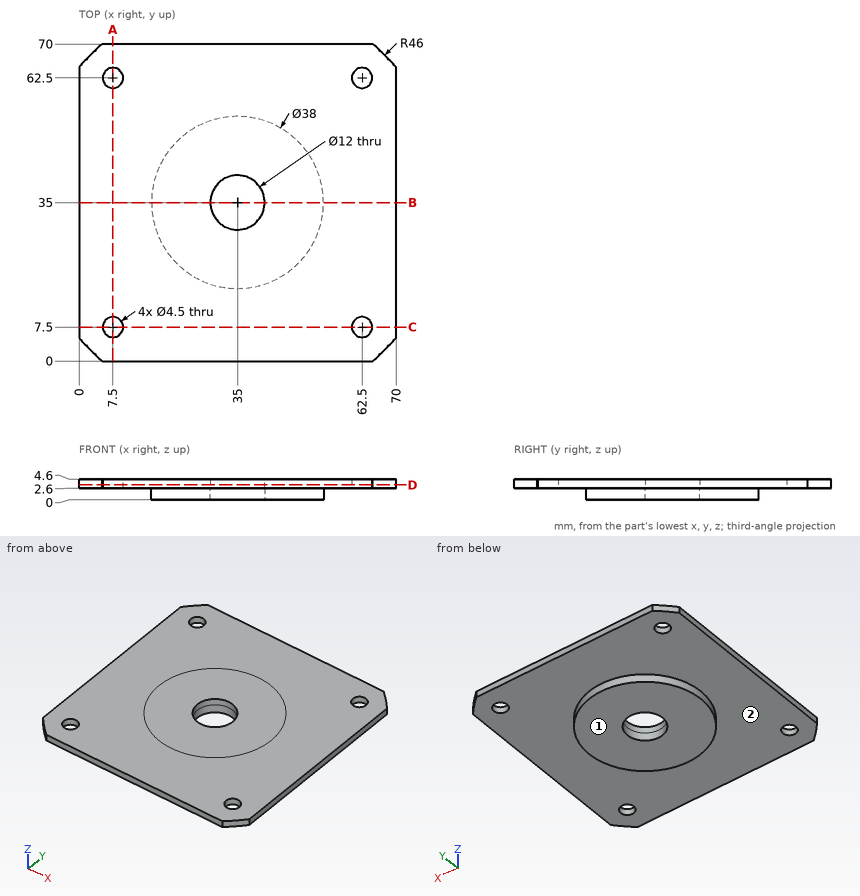
Design review of the part shown in the three views and the two pictorial views. Dimensions are in mm from the part's minimum x, y and z. A direction names the side the tool comes from. Round coordinates to 2 decimals unless told otherwise and drop trailing zeros. Write each loop counter-clockwise with the first axis right and the second up, starting at its lowest first coordinate (ties: lowest second). Pieces come first, ordered by that corner, then holes.
Item 1: Wall thickness on L1, parallel to Y at x = 7.5, z = 3.2; L2, parallel to Y at x = 35, z = 1.4; L3, parallel to Y at x = 35, z = 3.2: over which ranges is each line inside the solid? List them lowest first.
Item 2: Consider section D-D on z = 3.3. Give the boundary of the cut face in (x, y), and give its area (3 significant figures).
Item 3: For the marked faces 1 and 2, list the 3-axis set-ups (+Z, -Z, +X, -X, +Y, -Y) from which the entire face can be reached by the end or side of a thin tool; tool diameter is ignored.
Item 4: For pin 1 Ø11 at (x, y) = (35, 35) entering from +Z; pin 2 Ø2 at (x, y) = (24.5, 57.5) entering from -Z, all flat-tipped, find the tip position at first contact; note any pin that passes through.
Item 5: Consider section B-B on y = 35. Give the boundary of the cut face in (x, z).
Item 6: Consider section A-A on x = 7.5. Give the boundary of the cut face in (y, z), and give its area (3 significant figures).
Check values:
1. L1: y = 0 to 5.25, 9.75 to 60.25, 64.75 to 70
1. L2: y = 16 to 29, 41 to 54
1. L3: y = 0 to 29, 41 to 70
2. outline: (0, 5.15) arc R46 ccw to (5.15, 0) - (64.85, 0) arc R46 ccw to (70, 5.15) - (70, 64.85) arc R46 ccw to (64.85, 70) - (5.15, 70) arc R46 ccw to (0, 64.85) - close; hole circle Ø4.5 at (7.5, 7.5); hole circle Ø4.5 at (7.5, 62.5); hole circle Ø12 at (35, 35); hole circle Ø4.5 at (62.5, 7.5); hole circle Ø4.5 at (62.5, 62.5)
2. area: 4,670 mm2
3. face 1: -Z, +X, -X, +Y, -Y
3. face 2: -Z
4. pin 1: passes through
4. pin 2: stops at z = 2.6
5. outline: (0, 2.6) - (16, 2.6) - (16, 0) - (29, 0) - (29, 4.6) - (0, 4.6) - close; (41, 0) - (54, 0) - (54, 2.6) - (70, 2.6) - (70, 4.6) - (41, 4.6) - close
6. outline: (0, 2.6) - (5.25, 2.6) - (5.25, 4.6) - (0, 4.6) - close; (9.75, 2.6) - (60.25, 2.6) - (60.25, 4.6) - (9.75, 4.6) - close; (64.75, 2.6) - (70, 2.6) - (70, 4.6) - (64.75, 4.6) - close
6. area: 122 mm2
